Autodesk Fusion 360 part; units mm, degrees
sketch "Sketch1" plane through (0, 0, 0) normal (0, 1, 0) x (1, 0, 0)
  circle A0 centre (0, 0) radius 17
  circle A1 centre (0, 0) radius 14.895
  line L0 (0, 0) -> (0, 8) construction
  line L1 (0, 8) -> (2.5, 8)
  line L2 (2.5, 8) -> (2.5, 6.5383)
  line L3 (0, 8) -> (-2.5, 8)
  line L4 (-2.5, 8) -> (-2.5, 6.5383)
  arc A2 (-2.5, 6.5383) -> (2.5, 6.5383) centre (0, 0) ccw
  dimension "d1" = 34
  dimension "d2" = 29.79
  dimension "d3" = 14
  dimension "d4" = 2.5
  dimension "d5" = 2.5
  dimension "d6" = 8
extrude "Extrude1" add sketch "Sketch1" against normal blind 2.5 contours A0 | A1
extrude "Extrude2" add sketch "Sketch1" along normal blind 15 contours A1
extrude "Extrude3" add sketch "Sketch1" along normal blind 2.5 from surface at 15 contours A0 | A1
CAD build for the part. Positions are in the model's coordinates, mm. A direction names the side the tool comes from. Coordinates: 2 decimals unless noted, no trailing zeros. Write each loop counter-clockwise with the first axis right and the second up, starting at its lowest first coordinate (ties: lowest second). Pieces come first, ordered by that corner, then holes.
(1) 3-axis set-ups, long thin cutter, end or side, ignore diameter. For faces 1 (the face through (2.5, 7, -7)), 2 (the face through (1.2, 0, 15)), 3 (the face through (-0.2, -2.5, 7.3)): which of +Z, -Z, +X, -X, +Y, -Y reach the whole face in a straight line?
(2) Drill centre lines: probe 1 along Z at (x, y) = (0, 13) (3 decimals); probe 2 along X at (y, z) = (14.75, 0) (3 decimals); probe 3 along X at (y, z) = (16.5, 0). Where is each one in solid material? Low to high.
(3) Two-plate mould, pull along Z, no slides. Class faces 4 (the face through (-0.2, 17.5, 7.3)), 5 (the face through (0, 7, -8)), 6 (the face through (9.139, 16.233, 14.334)), 7 (the face through (0, 7, 7)): +Z half, -Z half, draft (parallel to the pull), parting line (faces both ways), or undercut.
(4) Cut at A-A, the plane z = 0. List the corners of the cut face in (x, y) (3 decimals).
(5) Flat gauge pins, fed straight in: pin 1 (6 mm diameter, centred on x = -3, y = 13.5, fed in from +Z); pin 2 (0.7 mm diameter, centred on y = 11.5, z = -7.5, fed in from +X); pin 3 (4 mm diameter, centred on y = 4, z = -1.5, fed in from -X) (3 decimals). Where does each tip first touch, or does it go through?
(6) Cut at C-C, the plane y = 1. List the corners of the cut face in (x, z) (3 decimals).
(7) Cut at D-D, the plane z = 8.5. List the corners of the cut face in (x, y).
(8) Cut at B-B, the plane x = 0. List the corners of the cut face in (y, z) (3 decimals), and give its area (3 significant figures).
Geometry says:
1. face 1: +Y, -Y
1. face 2: none
1. face 3: +Z, -Z, +X, -X, -Y
2. probe 1: z = -14.895 to -8, 7 to 14.895
2. probe 2: x = -14.895 to -7, 7 to 14.895
2. probe 3: x = -17 to -7, 7 to 17
3. face 4: draft
3. face 5: undercut
3. face 6: parting line
3. face 7: undercut
4. outline: (-17, -2.5) - (-7, -2.5) - (-7, 17.5) - (-17, 17.5) - (-17, 15) - (-14.895, 15) - (-14.895, 0) - (-17, 0) - close; (7, -2.5) - (17, -2.5) - (17, 0) - (14.895, 0) - (14.895, 15) - (17, 15) - (17, 17.5) - (7, 17.5) - close
5. pin 1: stops at z = 17
5. pin 2: stops at x = 13.07
5. pin 3: stops at x = -14.895
6. outline: circle Ø29.79 at (0, 0); hole (-2.5, -8) - (2.5, -8) - (2.5, -6.538) arc R7 ccw (long way) to (-2.5, -6.538) - close
7. outline: (-14.72, -2.5) - (14.72, -2.5) - (14.72, 0) - (12.23, 0) - (12.23, 15) - (14.72, 15) - (14.72, 17.5) - (-14.72, 17.5) - (-14.72, 15) - (-12.23, 15) - (-12.23, 0) - (-14.72, 0) - close
8. outline: (-2.5, -17) - (0, -17) - (0, -14.895) - (15, -14.895) - (15, -17) - (17.5, -17) - (17.5, -8) - (-2.5, -8) - close; (-2.5, 7) - (17.5, 7) - (17.5, 17) - (15, 17) - (15, 14.895) - (0, 14.895) - (0, 17) - (-2.5, 17) - close
8. area: 317 mm2
